from build123d import *

# Parameters (mm, degrees)
SKETCH1_R           = 2.5
BOSS_EXTRUDE1_DEPTH = 2


with BuildPart() as part:
    # Sketch1 → Boss-Extrude1 (new body)
    with BuildSketch(Plane.XY):
        with BuildLine():
            ThreePointArc((-95.826370741, 39.877946607), (-100.826370741, 34.877946607), (-95.826370741, 29.877946607))
            Line((-95.826370741, 29.877946607), (-65, 0))
            ThreePointArc((-65, 0), (-63.535533906, -3.535533906), (-60, -5))
            Line((-60, -5), (60, -5))
            ThreePointArc((60, -5), (63.535533906, -3.535533906), (65, 0))
            Line((65, 0), (95.826370741, 29.877946607))
            ThreePointArc((95.826370741, 29.877946607), (100.826370741, 34.877946607), (95.826370741, 39.877946607))
            Line((95.826370741, 39.877946607), (0, 49))
            Line((0, 49), (-95.826370741, 39.877946607))
        make_face()
        Circle(SKETCH1_R, mode=Mode.SUBTRACT)
        with Locations((-95.826370741, 34.877946607)):
            Circle(SKETCH1_R, mode=Mode.SUBTRACT)
        with Locations((0, 44)):
            Circle(SKETCH1_R, mode=Mode.SUBTRACT)
        with Locations((-60, 0)):
            Circle(SKETCH1_R, mode=Mode.SUBTRACT)
        with Locations((95.826370741, 34.877946607)):
            Circle(SKETCH1_R, mode=Mode.SUBTRACT)
        with Locations((60, 0)):
            Circle(SKETCH1_R, mode=Mode.SUBTRACT)
    extrude(amount=BOSS_EXTRUDE1_DEPTH)


solid = part.part
Verification items for the finished model (mm, model axes). Give positions to 0.01 mm unless a question says otherwise; leave off trailing zeros. Write each loop counter-clockwise with the first axis right and the second up, starting at its lowest first coordinate (ties: lowest second). Pieces come first, ordered by that corner, then holes.
(1) Cross-section at A-A (y = 44). Enter the section's corners in (x, z).
(2) Cross-section at B-B (z = 1.45). Enter the section's corners in (x, y).
(3) Gauge pin test, flat end, axial feed: pin 1 (1 mm diameter, centred on y = 34, z = 0.5, fed in from +X). Record the tip position at first contact, or that the pin passes through.
(4) Cross-section at C-C (x = 13.5). Enter the section's corners in (y, z), plus the area to 3 significant figures.
(5) Material ranges on line 1 (Y direction, x = 0, z = 1.35); line 2 (X direction, y = 36, z = 0.4); line 3 (X direction, y = -1, z = 1.65), recorded low to high.
(6) Mould release check, pull along Y, two halves, no side actions. Record for faces 1 (the face through (80.2, 14.73, 0.99)), 2 (the face through (48.584, 44.375, 0.986)), 3 (the face through (-57.69, -0.96, 0.99)), 4 (the face through (62.31, -0.96, 0.99)): +Y half, -Y half, draft (parallel to the pull), parting line (faces both ways), or undercut.
(7) Cross-section at D-D (y = 8). Enter the section's corners in (x, z), plus the area to 3 significant figures.
Worked out:
1. outline: (-52.52, 0) - (-2.5, 0) - (-2.5, 2) - (-52.52, 2) - close; (2.5, 0) - (52.52, 0) - (52.52, 2) - (2.5, 2) - close
2. outline: (-95.83, 29.88) - (-65, 0) arc R5 ccw to (-60, -5) - (60, -5) arc R5 ccw to (65, 0) - (95.83, 29.88) arc R5 ccw to (95.83, 39.88) - (0, 49) - (-95.83, 39.88) arc R5 ccw to start; hole circle Ø5 at (-95.83, 34.88); hole circle Ø5 at (-60, 0); hole circle Ø5 at (0, 0); hole circle Ø5 at (0, 44); hole circle Ø5 at (60, 0); hole circle Ø5 at (95.83, 34.88)
3. pin 1: stops at x = 100.81
4. outline: (-5, 0) - (47.71, 0) - (47.71, 2) - (-5, 2) - close
4. area: 105 mm2
5. line 1: y = -5 to -2.5, 2.5 to 41.5, 46.5 to 49
5. line 2: x = -100.7 to -98.06, -93.59 to 93.59, 98.06 to 100.7
5. line 3: x = -64.9 to -62.29, -57.71 to -2.29, 2.29 to 57.71, 62.29 to 64.9
6. face 1: -Y half
6. face 2: +Y half
6. face 3: undercut
6. face 4: undercut
7. outline: (-73.25, 0) - (73.25, 0) - (73.25, 2) - (-73.25, 2) - close
7. area: 293 mm2
